For this review, take the finished solid that the model builds, in its own axes (mm). A direction names the side the tool comes from. Coordinates: 2 decimals unless noted, no trailing zeros. Loops run counter-clockwise (first coordinate to the right, second up) from the corner with the lowest first, then second, coordinate; pieces in that order, holes last. Notation, with made-up numbers: (60.5, 52.5) - (86.5, 52.5) arc R37 ccw to (86.5, 91.5) - close; hole circle Ø7 at (-12.75, -33). An arc over 180 degrees is marked (long way). One line per item, written item: value. Start each with the question number.
1. Take a section at A-A, the plane x = 92.5. State the section outline as (y, z) points.
2. Take a section at C-C, the plane y = 51.5. Count the separate pieces of the cut face and the enclosed holes in it, and give its area (3 significant figures).
3. Take a section at B-B, the plane y = 183.5. State the section outline as (x, z) points.
4. For faces 1 (the face through (-2, 103, 174.523)), 2 (the face through (79.064, 24.84, -176.185)), 3 (the face through (-149.123, 103, 156)), list the 3-axis set-ups (+Z, -Z, +X, -X, +Y, -Y) from which the entire face can be reached by the end or side of a thin tool; tool diameter is ignored.
5. Take a section at D-D, the plane x = 48. State the section outline as (y, z) points, and give its area (3 significant figures).
6. The part is to be moulded in two halves that separate along Y. For faces 4 (the face through (150, 9.423, -164)), 5 (the face through (79.064, 171.807, -176.185)), 6 (the face through (-149.123, 106, -156)), say which applies: released by +Y, released by -Y, zero draft, split by the parting line, or undercut.
7. To check wall thickness, follow line 1 (Z direction, x = 44, y = 180); line 2 (X direction, y = 153, z = 144); line 3 (Y direction, x = -39.5, z = 118.5). State the ranges of each line that lie inside material, in increasing order. Write a range as from..to.
8. Insertion check: pin 1 (3.5 mm diameter, centred on y = 81, z = -176.5, fed in from -X); pin 2 (2.5 mm diameter, centred on x = -150.5, y = 116.5, fed in from -Z); pin 3 (3.5 mm diameter, centred on x = -119, y = -2.5, fed in from +Z). Each pin has a flat end and moves straight along its axis. Give the tip position at first contact, or say it passes through.
```python
from build123d import *

# Parameters (mm, degrees)
SKETCH1_W                       = 279.4
SKETCH1_H                       = 355.6
BASE_FLANGE1_DEPTH              = 3.2766
EDGE_FLANGE1_STRIP_W            = 18.42008
EDGE_FLANGE1_STRIP_H            = 3.2766
EDGE_FLANGE1_STRIP_CUT_DEPTH    = 279.4
EDGE_FLANGE1_STRIP_2_W          = 18.42008
EDGE_FLANGE1_STRIP_2_H          = 3.2766
EDGE_FLANGE1_STRIP_CUT_2_DEPTH  = 279.4
EDGE_FLANGE1_DEPTH              = 279.4
EDGE_FLANGE1_FLAT_DEPTH         = 3.2766
EDGE_FLANGE1_BEND_DEPTH         = 279.4
EDGE_FLANGE1_FLAT_2_DEPTH       = 3.2766
EDGE_FLANGE2_STRIP_W            = 18.42008
EDGE_FLANGE2_STRIP_H            = 3.2766
EDGE_FLANGE2_STRIP_CUT_DEPTH    = 190.5
EDGE_FLANGE2_STRIP_2_W          = 18.42008
EDGE_FLANGE2_STRIP_2_H          = 3.2766
EDGE_FLANGE2_STRIP_CUT_2_DEPTH  = 190.5
EDGE_FLANGE2_STRIP_3_W          = 18.42008
EDGE_FLANGE2_STRIP_3_H          = 3.2766
EDGE_FLANGE2_STRIP_CUT_3_DEPTH  = 190.5
EDGE_FLANGE2_STRIP_4_W          = 18.42008
EDGE_FLANGE2_STRIP_4_H          = 3.2766
EDGE_FLANGE2_STRIP_CUT_4_DEPTH  = 190.5
EDGE_FLANGE2_DEPTH              = 190.5
EDGE_FLANGE2_BEND_DEPTH         = 190.5
EDGE_FLANGE2_BEND_2_DEPTH       = 190.5
EDGE_FLANGE2_BEND_3_DEPTH       = 190.5
SKETCH34_W                      = 38.1
SKETCH34_H                      = 152.4
CUT_EXTRUDE1_DEPTH              = 436.484197035
FILLET1_R                       = 9.525
FILLET2_R                       = 3.175
F_1_4_START                     = -3.2766
F_1_4_0_25_DIAMETER_SLOT1_DEPTH = 3.2766
LPATTERN1_COUNT                 = 2
LPATTERN1_PITCH                 = 57.15
MIRROR1_START                   = -3.2766
MIRROR1_COPY_1_DEPTH            = 3.2766
F_1_4_0_25_DIAMETER_SLOT2_DEPTH = 3.2766


# Read off the part's stored shape, not the designer's step: 1/4 (0.25) Diameter Slot1, 1/4 (0.25) Diameter Slot2
# Sheet-metal steps are written as plain solids
with BuildPart() as part:
    # Sketch1 → Base-Flange1 (new body)
    with BuildSketch(Plane(origin=(0, 0, 0), x_dir=(1, 0, 0), z_dir=(0, 1, 0))):
        Rectangle(SKETCH1_W, SKETCH1_H)
    extrude(amount=-BASE_FLANGE1_DEPTH)

    # Edge-Flange1 strip (across the edge) → Edge-Flange1 strip cut (cut)
    with BuildSketch(Plane(origin=(-139.7, 0, 177.8), x_dir=(0, 0, -1), z_dir=(1, 0, 0))):
        with Locations((-3.2766, -1.6383)):
            Rectangle(EDGE_FLANGE1_STRIP_W, EDGE_FLANGE1_STRIP_H)
    extrude(amount=EDGE_FLANGE1_STRIP_CUT_DEPTH, mode=Mode.SUBTRACT)

    # Edge-Flange1 strip 2 (across the edge) → Edge-Flange1 strip cut 2 (cut)
    with BuildSketch(Plane(origin=(139.7, 0, -177.8), x_dir=(0, 0, 1), z_dir=(-1, 0, 0))):
        with Locations((-3.2766, -1.6383)):
            Rectangle(EDGE_FLANGE1_STRIP_2_W, EDGE_FLANGE1_STRIP_2_H)
    extrude(amount=EDGE_FLANGE1_STRIP_CUT_2_DEPTH, mode=Mode.SUBTRACT)

    # Edge-Flange1 bend section (across the edge) → Edge-Flange1 (add)
    with BuildSketch(Plane(origin=(-139.7, 0, 177.8), x_dir=(0, 0, -1), z_dir=(1, 0, 0))):
        with BuildLine():
            Line((0, 2.65684), (3.2766, 2.65684))
            ThreePointArc((3.2766, 2.65684), (4.054770419, 0.778170419), (5.93344, 0))
            Line((5.93344, 0), (5.93344, -3.2766))
            ThreePointArc((5.93344, -3.2766), (1.73786434, -1.53873566), (0, 2.65684))
        make_face()
    extrude(amount=EDGE_FLANGE1_DEPTH)

    # Edge-Flange1 profile (on flange) → Edge-Flange1 flat (add)
    with BuildSketch(Plane.XY.offset(177.8)):
        Polygon((-139.7, 2.65684), (139.7, 2.65684), (139.7, 9.4234), (152.4, 9.4234), (152.4, 199.9234), (-152.4, 199.9234), (-152.4, 9.4234), (-139.7, 9.4234), align=None)
    extrude(amount=-EDGE_FLANGE1_FLAT_DEPTH)

    # Edge-Flange1 bend section 2 (across the edge) → Edge-Flange1 bend (add)
    with BuildSketch(Plane(origin=(139.7, 0, -177.8), x_dir=(0, 0, 1), z_dir=(-1, 0, 0))):
        with BuildLine():
            Line((0, 2.65684), (3.2766, 2.65684))
            ThreePointArc((3.2766, 2.65684), (4.054770419, 0.778170419), (5.93344, 0))
            Line((5.93344, 0), (5.93344, -3.2766))
            ThreePointArc((5.93344, -3.2766), (1.73786434, -1.53873566), (0, 2.65684))
        make_face()
    extrude(amount=EDGE_FLANGE1_BEND_DEPTH)

    # Edge-Flange1 profile 2 (on flange) → Edge-Flange1 flat 2 (add)
    with BuildSketch(Plane(origin=(0, 0, -177.8), x_dir=(-1, 0, 0), z_dir=(0, 0, -1))):
        Polygon((-139.7, 9.4234), (-139.7, 2.65684), (139.7, 2.65684), (139.7, 9.4234), (152.4, 9.4234), (152.4, 199.9234), (-152.4, 199.9234), (-152.4, 9.4234), align=None)
    extrude(amount=-EDGE_FLANGE1_FLAT_2_DEPTH)

    # Edge-Flange2 strip (across the edge) → Edge-Flange2 strip cut (cut)
    with BuildSketch(Plane(origin=(-152.4, 9.4234, 174.5234), x_dir=(1, 0, 0), z_dir=(0, 1, 0))):
        with Locations((-3.2766, -1.6383)):
            Rectangle(EDGE_FLANGE2_STRIP_W, EDGE_FLANGE2_STRIP_H)
    extrude(amount=EDGE_FLANGE2_STRIP_CUT_DEPTH, mode=Mode.SUBTRACT)

    # Edge-Flange2 strip 2 (across the edge) → Edge-Flange2 strip cut 2 (cut)
    with BuildSketch(Plane(origin=(152.4, 199.9234, 174.5234), x_dir=(-1, 0, 0), z_dir=(0, -1, 0))):
        with Locations((-3.2766, -1.6383)):
            Rectangle(EDGE_FLANGE2_STRIP_2_W, EDGE_FLANGE2_STRIP_2_H)
    extrude(amount=EDGE_FLANGE2_STRIP_CUT_2_DEPTH, mode=Mode.SUBTRACT)

    # Edge-Flange2 strip 3 (across the edge) → Edge-Flange2 strip cut 3 (cut)
    with BuildSketch(Plane(origin=(-152.4, 199.9234, -174.5234), x_dir=(1, 0, 0), z_dir=(0, -1, 0))):
        with Locations((-3.2766, -1.6383)):
            Rectangle(EDGE_FLANGE2_STRIP_3_W, EDGE_FLANGE2_STRIP_3_H)
    extrude(amount=EDGE_FLANGE2_STRIP_CUT_3_DEPTH, mode=Mode.SUBTRACT)

    # Edge-Flange2 strip 4 (across the edge) → Edge-Flange2 strip cut 4 (cut)
    with BuildSketch(Plane(origin=(152.4, 9.4234, -174.5234), x_dir=(-1, 0, 0), z_dir=(0, 1, 0))):
        with Locations((-3.2766, -1.6383)):
            Rectangle(EDGE_FLANGE2_STRIP_4_W, EDGE_FLANGE2_STRIP_4_H)
    extrude(amount=EDGE_FLANGE2_STRIP_CUT_4_DEPTH, mode=Mode.SUBTRACT)

    # Edge-Flange2 section (across the edge) → Edge-Flange2 (add)
    with BuildSketch(Plane(origin=(-152.4, 9.4234, 174.5234), x_dir=(1, 0, 0), z_dir=(0, 1, 0))):
        with BuildLine():
            Line((0, 2.65684), (0, 34.8234))
            Line((0, 34.8234), (3.2766, 34.8234))
            Line((3.2766, 34.8234), (3.2766, 2.65684))
            ThreePointArc((3.2766, 2.65684), (4.054770419, 0.778170419), (5.93344, 0))
            Line((5.93344, 0), (5.93344, -3.2766))
            ThreePointArc((5.93344, -3.2766), (1.73786434, -1.53873566), (0, 2.65684))
        make_face()
    extrude(amount=EDGE_FLANGE2_DEPTH)

    # Edge-Flange2 section 2 (across the edge) → Edge-Flange2 bend (add)
    with BuildSketch(Plane(origin=(152.4, 199.9234, 174.5234), x_dir=(-1, 0, 0), z_dir=(0, -1, 0))):
        with BuildLine():
            Line((0, 2.65684), (0, 34.8234))
            Line((0, 34.8234), (3.2766, 34.8234))
            Line((3.2766, 34.8234), (3.2766, 2.65684))
            ThreePointArc((3.2766, 2.65684), (4.054770419, 0.778170419), (5.93344, 0))
            Line((5.93344, 0), (5.93344, -3.2766))
            ThreePointArc((5.93344, -3.2766), (1.73786434, -1.53873566), (0, 2.65684))
        make_face()
    extrude(amount=EDGE_FLANGE2_BEND_DEPTH)

    # Edge-Flange2 section 3 (across the edge) → Edge-Flange2 bend 2 (add)
    with BuildSketch(Plane(origin=(-152.4, 199.9234, -174.5234), x_dir=(1, 0, 0), z_dir=(0, -1, 0))):
        with BuildLine():
            Line((0, 2.65684), (0, 34.8234))
            Line((0, 34.8234), (3.2766, 34.8234))
            Line((3.2766, 34.8234), (3.2766, 2.65684))
            ThreePointArc((3.2766, 2.65684), (4.054770419, 0.778170419), (5.93344, 0))
            Line((5.93344, 0), (5.93344, -3.2766))
            ThreePointArc((5.93344, -3.2766), (1.73786434, -1.53873566), (0, 2.65684))
        make_face()
    extrude(amount=EDGE_FLANGE2_BEND_2_DEPTH)

    # Edge-Flange2 section 4 (across the edge) → Edge-Flange2 bend 3 (add)
    with BuildSketch(Plane(origin=(152.4, 9.4234, -174.5234), x_dir=(-1, 0, 0), z_dir=(0, 1, 0))):
        with BuildLine():
            Line((0, 2.65684), (0, 34.8234))
            Line((0, 34.8234), (3.2766, 34.8234))
            Line((3.2766, 34.8234), (3.2766, 2.65684))
            ThreePointArc((3.2766, 2.65684), (4.054770419, 0.778170419), (5.93344, 0))
            Line((5.93344, 0), (5.93344, -3.2766))
            ThreePointArc((5.93344, -3.2766), (1.73786434, -1.53873566), (0, 2.65684))
        make_face()
    extrude(amount=EDGE_FLANGE2_BEND_3_DEPTH)

    # Sketch34 → Cut-Extrude1 (cut, through all)
    with BuildSketch(Plane.XY.offset(177.8)):
        with Locations((-95.25, 98.3234)):
            Rectangle(SKETCH34_W, SKETCH34_H)
        with Locations((95.25, 98.3234)):
            Rectangle(SKETCH34_W, SKETCH34_H)
    extrude(amount=-CUT_EXTRUDE1_DEPTH, mode=Mode.SUBTRACT)

    # Fillet1
    fillet1_edges = [part.edges().sort_by_distance(p)[0] for p in [
        (-76.2, 174.5234, -176.1617),
        (-76.2, 22.1234, -176.1617),
        (-114.3, 22.1234, -176.1617),
        (-114.3, 174.5234, -176.1617),
        (-76.2, 174.5234, 176.1617),
        (-76.2, 22.1234, 176.1617),
        (-114.3, 22.1234, 176.1617),
        (-114.3, 174.5234, 176.1617),
        (76.2, 22.1234, -176.1617),
        (76.2, 174.5234, -176.1617),
        (114.3, 174.5234, -176.1617),
        (114.3, 22.1234, -176.1617),
        (76.2, 22.1234, 176.1617),
        (76.2, 174.5234, 176.1617),
        (114.3, 174.5234, 176.1617),
        (114.3, 22.1234, 176.1617),
    ]]
    fillet(fillet1_edges, radius=FILLET1_R)

    # Fillet2
    fillet2_edges = [part.edges().sort_by_distance(p)[0] for p in [
        (-150.7617, 9.4234, 139.7),
        (-150.7617, 199.9234, 139.7),
        (150.7617, 199.9234, 139.7),
        (150.7617, 9.4234, 139.7),
        (-150.7617, 199.9234, -139.7),
        (-150.7617, 9.4234, -139.7),
        (150.7617, 9.4234, -139.7),
        (150.7617, 199.9234, -139.7),
        (-139.7, 9.4234, 176.1617),
        (139.7, 9.4234, 176.1617),
        (139.7, 9.4234, -176.1617),
        (-139.7, 9.4234, -176.1617),
    ]]
    fillet(fillet2_edges, radius=FILLET2_R)

    # 1/4 (0.25) Diameter Slot1 outline → 1/4 (0.25) Diameter Slot1 (cut)
    with BuildSketch(Plane(origin=(0, 0, 0), x_dir=(1, 0, 0), z_dir=(0, 1, 0)).offset(F_1_4_START)):
        with BuildLine():
            ThreePointArc((-114.3, 152.4), (-111.125, 155.575), (-114.3, 158.75))
            Line((-114.3, 158.75), (-127, 158.75))
            ThreePointArc((-127, 158.75), (-130.175, 155.575), (-127, 152.4))
            Line((-127, 152.4), (-114.3, 152.4))
        make_face()
        with BuildLine():
            ThreePointArc((114.3, 158.75), (111.125, 155.575), (114.3, 152.4))
            Line((114.3, 152.4), (127, 152.4))
            ThreePointArc((127, 152.4), (130.175, 155.575), (127, 158.75))
            Line((127, 158.75), (114.3, 158.75))
        make_face()
    f_1_4_0_25_diameter_slot1 = extrude(amount=F_1_4_0_25_DIAMETER_SLOT1_DEPTH, mode=Mode.SUBTRACT)

    # LPattern1: 1/4 (0.25) Diameter Slot1 ×2
    with Locations(*[(0, 0, i * LPATTERN1_PITCH) for i in range(1, LPATTERN1_COUNT)]):
        add(f_1_4_0_25_diameter_slot1, mode=Mode.SUBTRACT)

    # Mirror1: 1/4 (0.25) Diameter Slot1 across plane
    add(f_1_4_0_25_diameter_slot1.mirror(Plane.XY), mode=Mode.SUBTRACT)

    # Mirror1 copy 1 sketch → Mirror1 copy 1 (cut)
    with BuildSketch(Plane(origin=(0, 0, -57.15), x_dir=(1, 0, 0), z_dir=(0, 1, 0)).offset(MIRROR1_START)):
        with BuildLine():
            ThreePointArc((-114.3, -152.4), (-111.125, -155.575), (-114.3, -158.75))
            Line((-114.3, -158.75), (-127, -158.75))
            ThreePointArc((-127, -158.75), (-130.175, -155.575), (-127, -152.4))
            Line((-127, -152.4), (-114.3, -152.4))
        make_face()
        with BuildLine():
            ThreePointArc((114.3, -158.75), (111.125, -155.575), (114.3, -152.4))
            Line((114.3, -152.4), (127, -152.4))
            ThreePointArc((127, -152.4), (130.175, -155.575), (127, -158.75))
            Line((127, -158.75), (114.3, -158.75))
        make_face()
    extrude(amount=MIRROR1_COPY_1_DEPTH, mode=Mode.SUBTRACT)

    # 1/4 (0.25) Diameter Slot2 outline → 1/4 (0.25) Diameter Slot2 (cut)
    with BuildSketch(Plane(origin=(0, 0, 0), x_dir=(1, 0, 0), z_dir=(0, 1, 0)).offset(F_1_4_START)):
        with BuildLine():
            ThreePointArc((-120.65, 6.35), (-123.825, 9.525), (-127, 6.35))
            Line((-127, 6.35), (-127, -6.35))
            ThreePointArc((-127, -6.35), (-123.825, -9.525), (-120.65, -6.35))
            Line((-120.65, -6.35), (-120.65, 6.35))
        make_face()
        with BuildLine():
            ThreePointArc((127, 6.35), (123.825, 9.525), (120.65, 6.35))
            Line((120.65, 6.35), (120.65, -6.35))
            ThreePointArc((120.65, -6.35), (123.825, -9.525), (127, -6.35))
            Line((127, -6.35), (127, 6.35))
        make_face()
    extrude(amount=F_1_4_0_25_DIAMETER_SLOT2_DEPTH, mode=Mode.SUBTRACT)


solid = part.part
```
Solutions:
1. outline: (-3.28, -171.87) arc R5.93 ccw to (2.66, -177.8) - (22.12, -177.8) - (22.12, -174.52) - (2.66, -174.52) arc R2.66 cw to (0, -171.87) - (0, 171.87) arc R2.66 cw to (2.66, 174.52) - (22.12, 174.52) - (22.12, 177.8) - (2.66, 177.8) arc R5.93 ccw to (-3.28, 171.87) - close; (174.52, -177.8) - (199.92, -177.8) - (199.92, -174.52) - (174.52, -174.52) - close; (174.52, 174.52) - (199.92, 174.52) - (199.92, 177.8) - (174.52, 177.8) - close
2. separate pieces: 6
2. enclosed holes: 0
2. area: 1,930 mm2
3. outline: (-152.4, -171.87) arc R5.93 ccw to (-146.47, -177.8) - (146.47, -177.8) arc R5.93 ccw to (152.4, -171.87) - (152.4, -139.7) - (149.12, -139.7) - (149.12, -171.87) arc R2.66 cw to (146.47, -174.52) - (-146.47, -174.52) arc R2.66 cw to (-149.12, -171.87) - (-149.12, -139.7) - (-152.4, -139.7) - close; (-152.4, 139.7) - (-149.12, 139.7) - (-149.12, 171.87) arc R2.66 cw to (-146.47, 174.52) - (146.47, 174.52) arc R2.66 cw to (149.12, 171.87) - (149.12, 139.7) - (152.4, 139.7) - (152.4, 171.87) arc R5.93 ccw to (146.47, 177.8) - (-146.47, 177.8) arc R5.93 ccw to (-152.4, 171.87) - close
4. face 1: +Y
4. face 2: +Z, -Z
4. face 3: +Y, -Y
5. outline: (-3.28, -171.87) arc R5.93 ccw to (2.66, -177.8) - (199.92, -177.8) - (199.92, -174.52) - (2.66, -174.52) arc R2.66 cw to (0, -171.87) - (0, 171.87) arc R2.66 cw to (2.66, 174.52) - (199.92, 174.52) - (199.92, 177.8) - (2.66, 177.8) arc R5.93 ccw to (-3.28, 171.87) - close
5. area: 2,460 mm2
6. face 4: released by -Y
6. face 5: undercut
6. face 6: zero draft
7. line 1: -177.8..-174.52, 174.52..177.8
7. line 2: -152.4..-149.12, 149.12..152.4
7. line 3: -3.28..0
8. pin 1: x = -151.65
8. pin 2: z = -177.11
8. pin 3: z = 176.72
